```python
from build123d import *

# Parameters (mm, degrees)
F0_W     = 10.5
F0_H     = 12.5
F0_R     = 1.575
F1_DEPTH = 2
F2_SIZE  = 0.75


with BuildPart() as f1:
    # F0 (on Top) → F1 (new body)
    with BuildSketch(Plane.XY):
        Rectangle(F0_W, F0_H)
        with Locations((-2.5, -3.9)):
            Circle(F0_R, mode=Mode.SUBTRACT)
        with Locations((2.5, -3.9)):
            Circle(F0_R, mode=Mode.SUBTRACT)
        with Locations((-2.5, 0)):
            Circle(F0_R, mode=Mode.SUBTRACT)
        with Locations((-2.5, 3.9)):
            Circle(F0_R, mode=Mode.SUBTRACT)
        with Locations((2.5, 0)):
            Circle(F0_R, mode=Mode.SUBTRACT)
        with Locations((2.5, 3.9)):
            Circle(F0_R, mode=Mode.SUBTRACT)
    extrude(amount=F1_DEPTH)

    # F2
    f2_edges = [f1.edges().sort_by_distance(p)[0] for p in [
        (-5.25, 6.25, 1),
        (5.25, 6.25, 1),
        (5.25, -6.25, 1),
        (-5.25, -6.25, 1),
    ]]
    chamfer(f2_edges, length=F2_SIZE)


solid = f1.part
```
Here's how the part is built. I have some questions about the finished solid (model axes, mm). Give positions to 0.01 mm unless a question says otherwise; leave off trailing zeros. Write each loop counter-clockwise with the first axis right and the second up, starting at its lowest first coordinate (ties: lowest second). Pieces come first, ordered by that corner, then holes.
(1) Thinking about a two-plate mould opening in Y: for faces 1 (the face through (4.002, 0.473, 0.986)), 2 (the face through (0, -6.25, 1)), 3 (the face through (5.25, 0, 1)), 4 (the face through (3.347, 5.228, 0.986)), which applies, pulls with the +Y half, pulls with the -Y half, needs draft (parallel to the pull), parting line crosses it, or undercut?
Output values:
face 1: undercut
face 2: pulls with the -Y half
face 3: needs draft
face 4: undercut
(2) Imagine slicing it at B-B, the plane x = -2.5. Write out the boundary of the cut face in (y, z) (3 decimals).
Output values:
outline: (-6.25, 0) - (-5.475, 0) - (-5.475, 2) - (-6.25, 2) - close; (-2.325, 0) - (-1.575, 0) - (-1.575, 2) - (-2.325, 2) - close; (1.575, 0) - (2.325, 0) - (2.325, 2) - (1.575, 2) - close; (5.475, 0) - (6.25, 0) - (6.25, 2) - (5.475, 2) - close
(3) Will these pins go through, and if not, where does the flat tip stop? pin 1 (3.5 mm diameter, centred on x = 2.5, y = 0, fed in from -Z); pin 2 (2.5 mm diameter, centred on x = 2.5, y = 3.9, fed in from +Z).
Output values:
pin 1: stops at z = 0
pin 2: passes through
(4) Imagine slicing it at D-D, the plane y = 1. Write out the boundary of the cut face in (x, z), and give its area (3 significant figures).
Output values:
outline: (-5.25, 0) - (-3.72, 0) - (-3.72, 2) - (-5.25, 2) - close; (-1.28, 0) - (1.28, 0) - (1.28, 2) - (-1.28, 2) - close; (3.72, 0) - (5.25, 0) - (5.25, 2) - (3.72, 2) - close
area: 11.3 mm2
(5) If I drill on L1, parallel to Y at x = 2.5, z = 0.6 (3 decimals); L2, parallel to Y at x = 2, z = 1.35; L3, parallel to X at y = 3.25, z = 1.6, over which ranges is the centre line in solid material (lowest first)?
Output values:
L1: y = -6.25 to -5.475, -2.325 to -1.575, 1.575 to 2.325, 5.475 to 6.25
L2: y = -6.25 to -5.39, -2.41 to -1.49, 1.49 to 2.41, 5.39 to 6.25
L3: x = -5.25 to -3.93, -1.07 to 1.07, 3.93 to 5.25
(6) Imagine slicing it at A-A, the plane z = 0.15. Write out the boundary of the cut face in (x, y) (3 decimals), and give its area (3 significant figures).
Output values:
outline: (-5.25, -5.5) - (-4.5, -6.25) - (4.5, -6.25) - (5.25, -5.5) - (5.25, 5.5) - (4.5, 6.25) - (-4.5, 6.25) - (-5.25, 5.5) - close; hole circle Ø3.15 at (-2.5, -3.9); hole circle Ø3.15 at (-2.5, 0); hole circle Ø3.15 at (-2.5, 3.9); hole circle Ø3.15 at (2.5, -3.9); hole circle Ø3.15 at (2.5, 0); hole circle Ø3.15 at (2.5, 3.9)
area: 83.4 mm2
(7) Imagine slicing it at C-C, the plane y = 3.9. Write out the boundary of the cut face in (x, z) (3 decimals).
Output values:
outline: (-5.25, 0) - (-4.075, 0) - (-4.075, 2) - (-5.25, 2) - close; (-0.925, 0) - (0.925, 0) - (0.925, 2) - (-0.925, 2) - close; (4.075, 0) - (5.25, 0) - (5.25, 2) - (4.075, 2) - close
